```python
from build123d import *

# Parameters (mm, degrees)
BOSS_EXTRUDE1_DEPTH = 12
BOSS_EXTRUDE2_DEPTH = 2
CUT_EXTRUDE1_DEPTH  = 10
FILLET1_R           = 0.4


with BuildPart() as part:
    # Sketch1 → Boss-Extrude1 (new body)
    with BuildSketch(Plane(origin=(0, 0, 0), x_dir=(1, 0, 0), z_dir=(0, 1, 0))):
        with BuildLine():
            Line((-1.7, -2.471841419), (-1.7, -5.754128952))
            ThreePointArc((-1.7, -5.754128952), (0, 6), (1.7, -5.754128952))
            Line((1.7, -5.754128952), (1.7, -2.471841419))
            ThreePointArc((1.7, -2.471841419), (0, 3), (-1.7, -2.471841419))
        make_face()
    extrude(amount=BOSS_EXTRUDE1_DEPTH)

    # Sketch2 → Boss-Extrude2 (add)
    with BuildSketch(Plane.XZ):
        with BuildLine():
            Line((-1.7, 5.754128952), (-1.7, 9.854440623))
            ThreePointArc((-1.7, 9.854440623), (0, -10), (1.7, 9.854440623))
            Line((1.7, 9.854440623), (1.7, 5.754128952))
            ThreePointArc((1.7, 5.754128952), (0, -6), (-1.7, 5.754128952))
        make_face()
    extrude(amount=-BOSS_EXTRUDE2_DEPTH)

    # Sketch3 → Cut-Extrude1 (cut)
    with BuildSketch(Plane(origin=(0, 12, 0), x_dir=(1, 0, 0), z_dir=(0, 1, 0))):
        with BuildLine():
            Line((-0.75, 5.95294045), (-0.75, 5))
            Line((-0.75, 5), (0.75, 5))
            Line((0.75, 5), (0.75, 5.95294045))
            ThreePointArc((0.75, 5.95294045), (0, 6), (-0.75, 5.95294045))
        make_face()
    extrude(amount=-CUT_EXTRUDE1_DEPTH, mode=Mode.SUBTRACT)

    # Fillet1
    fillet1_edges = [part.edges().sort_by_distance(p)[0] for p in [
        (-0.75, 7, -5),
        (0.75, 7, -5),
    ]]
    fillet(fillet1_edges, radius=FILLET1_R)


solid = part.part
```
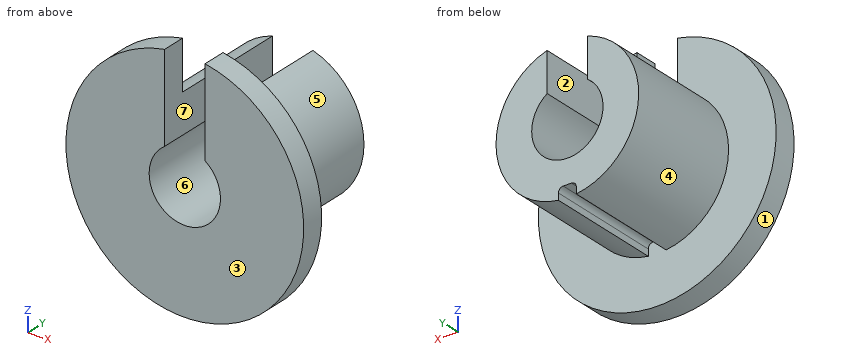
Verification items for the finished model (mm, model axes). Face numbers are marked on the shaded views. A direction names the side the tool comes from. Coordinates: 2 decimals unless noted, no trailing zeros. Loops run counter-clockwise (first coordinate to the right, second up) from the corner with the lowest first, then second, coordinate; pieces in that order, holes last. Notation, with made-up numbers: (7.5, 81.25) -> (21.5, 81.25) arc R18 cw to (21.5, 105.25) -> close; hole circle Ø11 at (22.25, 0). An arc over 180 degrees is marked (long way). Answer in a Markdown table with one row per item. Add a question column.
1. Section check D-D, the plane z = 3.75. Enter the section's corners in (x, y).
2. Section check A-A, the plane z = 0. Enter the section's corners in (x, y).
3. Access from +Z, -Z, +X, -X, +Y, -Y to the whole of each face (thin tool, end or side, straight path). Record for the marked faces 4, 5, 6 and 7.
4. Section check B-B, the plane x = 0. Enter the section's corners in (y, z).
5. Material ranges on probe 1 along X at (y, z) = (9.5, 0); probe 2 along X at (y, z) = (11.5, 3.25); probe 3 along Y at (x, z) = (7.75, 3.25), recorded low to high. Write a range as [from, to].
6. Section check C-C, the plane y = 10.25. Enter the section's corners in (x, z).
7. Draft check along X on the marked faces 1, 2 and 3. Enter one of: +X half, -X half, draft (parallel to the pull), parting line (faces both ways), or undercut.
8. Depth check by flat-ended pin: P1, Ø4, axis at y = 1.5, z = -8, coming from the +X side; P2, Ø4, axis at y = 1.5, z = -8, coming from the -X side; P3, Ø3, axis at x = -5, y = 2, coming from the -Z side. Enter the tip coordinate at first touch or a pass-through.
Derived:
| question | item | result |
|---|---|---|
| 1 | outline | (-9.27, 0) -> (-1.7, 0) -> (-1.7, 12) -> (-4.68, 12) -> (-4.68, 2) -> (-9.27, 2) -> close; (1.7, 0) -> (9.27, 0) -> (9.27, 2) -> (4.68, 2) -> (4.68, 12) -> (1.7, 12) -> close |
| 2 | outline | (-10, 0) -> (-3, 0) -> (-3, 12) -> (-6, 12) -> (-6, 2) -> (-10, 2) -> close; (3, 0) -> (10, 0) -> (10, 2) -> (6, 2) -> (6, 12) -> (3, 12) -> close |
| 3 | face 4 | -X, +Y |
| 3 | face 5 | +X, +Y |
| 3 | face 6 | +Y, -Y |
| 3 | face 7 | +Z, +Y, -Y |
| 4 | outline | (0, -10) -> (2, -10) -> (2, -5) -> (12, -5) -> (12, -3) -> (0, -3) -> close |
| 5 | probe 1 | x = [-6, -3], [3, 6] |
| 5 | probe 2 | x = [-5.04, -1.7], [1.7, 5.04] |
| 5 | probe 3 | y = [0, 2] |
| 6 | outline | (-1.7, 2.47) -> (-1.7, 5.75) arc R6 ccw to (-0.75, -5.95) -> (-0.75, -5.4) arc R0.4 cw to (-0.35, -5) -> (0.35, -5) arc R0.4 cw to (0.75, -5.4) -> (0.75, -5.95) arc R6 ccw to (1.7, 5.75) -> (1.7, 2.47) arc R3 cw (long way) to start |
| 7 | face 1 | parting line |
| 7 | face 2 | undercut |
| 7 | face 3 | draft |
| 8 | P1 | stops at x = 8 |
| 8 | P2 | stops at x = -8 |
| 8 | P3 | stops at z = -9.37 |
